Could you check a few things on this model? Use its own coordinates, in mm. A direction names the side the tool comes from. Give positions to 0.01 mm unless a question says otherwise; leave off trailing zeros. Write each loop counter-clockwise with the first axis right and the second up, starting at its lowest first coordinate (ties: lowest second). Pieces come first, ordered by that corner, then holes. Notation, with made-up numbers: (15.5, -17.75) -> (27.5, -17.75) arc R15 ccw to (27.5, 5.25) -> close; hole circle Ø4 at (-14, 5). An arc over 180 degrees is marked (long way). One line per question, with ' | ' between items.
from build123d import *

# Parameters (mm, degrees)
F0_W      = 81.613116
F0_H      = 28.127378
F1_DEPTH  = 12.192
F2_W      = 81.937075
F2_H      = 6.007762
F3_DEPTH  = 5.842
F4_W      = 81.90459
F4_H      = 5.975246
F5_DEPTH  = 19.05
F6_W      = 81.61312
F6_H      = 6.120986
F7_DEPTH  = 6.604
F8_R      = 5.659431
F8_R_2    = 6.127921
F9_DEPTH  = 70.104
F10_W     = 35.560001
F10_H     = 7.578362
F11_DEPTH = 5.08


with BuildPart() as f1:
    # F0 (on Front) → F1 (new body)
    with BuildSketch(Plane.XZ):
        with Locations((5.246557, 14.063689)):
            Rectangle(F0_W, F0_H)
    extrude(amount=F1_DEPTH)

    # F2 (on Front) → F3 (join)
    with BuildSketch(Plane.XZ):
        with Locations((5.226239, 3.003881)):
            Rectangle(F2_W, F2_H)
    extrude(amount=-F3_DEPTH)

    # F4 (on Front) → F5 (join)
    with BuildSketch(Plane.XZ):
        with Locations((5.10082, 2.987623)):
            Rectangle(F4_W, F4_H)
    extrude(amount=F5_DEPTH)

    # F6 (on Front) → F7 (join)
    with BuildSketch(Plane.XZ):
        with Locations((4.955081, 24.775409)):
            Rectangle(F6_W, F6_H)
    extrude(amount=-F7_DEPTH)

    # F8 (on face) → F9 (cut)
    with BuildSketch(Plane(origin=(0, 0, 0), x_dir=(-1, 0, 0), z_dir=(0, 1, 0))):
        with Locations((-30.604918, 14.428033)):
            Circle(F8_R)
        with Locations((16.6141, 13.553606)):
            Circle(F8_R_2)
    extrude(amount=-F9_DEPTH, mode=Mode.SUBTRACT)

    # F10 (on face) → F11 (join)
    with BuildSketch(Plane.XZ.offset(12.192)):
        with Locations((-17.78, 24.338197)):
            Rectangle(F10_W, F10_H)
    extrude(amount=F11_DEPTH)


solid = f1.part
Q1. On a 3-axis mill with a long thin cutter (end or side, diameter ignored), from which of +Z, -Z, +X, -X, +Y, -Y can I reach the whole of each face in a straight line? I mean faces 1 (the flat face through (45.762, 3, 25)), 2 (the flat face through (0, -15, 24)), 3 (the flat face through (-35.742, 3, 3)), 4 (the flat face through (5, 5.842, 3)), 5 (the flat face through (-35.56, -15, 24)). Say none if no direction works.
Answer below:
face 1: +Z, +X, +Y | face 2: +Z, +X, -Y | face 3: -Z, -X, +Y | face 4: -Z, +X, -X, +Y | face 5: +Z, -X, -Y
Q2. Imagine slicing it at D-D on x = -11.5. Please give me the cut outline in (y, z).
Answer below:
outline: (-19.05, 0) -> (5.84, 0) -> (5.84, 6.01) -> (0, 6.01) -> (0, 10.18) -> (-12.19, 10.18) -> (-12.19, 5.98) -> (-19.05, 5.98) -> close; (-17.27, 20.55) -> (-12.19, 20.55) -> (-12.19, 16.93) -> (0, 16.93) -> (0, 21.71) -> (6.6, 21.71) -> (6.6, 27.84) -> (0, 27.84) -> (0, 28.13) -> (-17.27, 28.13) -> close
Q3. If I drill on line 1 along Z through (x, y) = (30.5, -8.25); line 2 along X through (y, z) = (-4.5, 10); line 3 along Z through (x, y) = (-16, -15), over which ranges is the centre line in solid material (lowest first)?
Answer below:
line 1: z = 0 to 8.77, 20.09 to 28.13 | line 2: x = -35.56 to -21.61, -11.62 to 27.08, 34.13 to 46.05 | line 3: z = 0 to 5.98, 20.55 to 28.13
Q4. Imagine slicing it at C-C on z = 18. Please give me the cut outline in (x, y).
Answer below:
outline: (-35.56, -12.19) -> (-20.83, -12.19) -> (-20.83, 0) -> (-35.56, 0) -> close; (-12.4, -12.19) -> (26.22, -12.19) -> (26.22, 0) -> (-12.4, 0) -> close; (34.99, -12.19) -> (46.05, -12.19) -> (46.05, 0) -> (34.99, 0) -> close
Q5. If we mould it in two halves opening along Z, with no side actions, what happens to faces 6 (the flat face through (5, -6, 0)), 7 (the flat face through (46.053, -7, 14)), 8 (the flat face through (4, 3, 27.836)), 9 (the flat face through (5, -14, 5.975))? For each: +Z half, -Z half, draft (parallel to the pull), parting line (faces both ways), or undercut.
Answer below:
face 6: -Z half | face 7: draft | face 8: +Z half | face 9: undercut
Q6. Imagine slicing it at B-B on x = 2. Please give me the cut outline in (y, z).
Answer below:
outline: (-19.05, 0) -> (5.84, 0) -> (5.84, 6.01) -> (0, 6.01) -> (0, 21.71) -> (6.6, 21.71) -> (6.6, 27.84) -> (0, 27.84) -> (0, 28.13) -> (-12.19, 28.13) -> (-12.19, 5.98) -> (-19.05, 5.98) -> close
Q7. Imagine slicing it at A-A on y = 1.5. Please give me the cut outline in (x, z).
Answer below:
outline: (-35.85, 21.71) -> (45.76, 21.71) -> (45.76, 27.84) -> (-35.85, 27.84) -> close; (-35.74, 0) -> (46.19, 0) -> (46.19, 6.01) -> (-35.74, 6.01) -> close
Q8. Will these pins go through, and if not, where does the flat tip stop? pin 1 (8 mm diameter, centred on x = -23.5, z = 18.5, fed in from -Y); pin 2 (11 mm diameter, centred on x = 3.5, z = 12.5, fed in from -Y); pin 3 (12 mm diameter, centred on y = -13.5, z = 12.5, fed in from +X); pin 4 (7.5 mm diameter, centred on x = -11.5, y = 3.5, fed in from -Z).
Answer below:
pin 1: stops at y = -17.27 | pin 2: stops at y = -12.19 | pin 3: stops at x = 46.05 | pin 4: stops at z = 0
